For this review, take the finished solid that the model builds, in its own axes (mm). A direction names the side the tool comes from. Coordinates: 2 decimals unless noted, no trailing zeros. Write each loop counter-clockwise with the first axis right and the second up, starting at its lowest first coordinate (ties: lowest second). Pieces come first, ordered by that corner, then holes. Notation, with made-up numbers: (-34.5, 14.25) -> (19.5, 14.25) arc R17 cw to (19.5, 27.25) -> close; hole circle Ø1 at (73, 66.5). An arc over 180 degrees is marked (long way). Put each result on its own line as item: value. Start each with the question number.
Item 1: For faces 5 (the cylindrical face through (247.2, -3.47, -15.62)), 6 (the cylindrical face through (109, -6, 0)), list the 3-axis set-ups (+Z, -Z, +X, -X, +Y, -Y) from which the entire face can be reached by the end or side of a thin tool; tool diameter is ignored.
Item 2: Consider section C-C on y = -11. Give the boundary of the cut face in (x, z), and give its area (3 significant figures).
Item 3: Consider section A-A on z = 0. Give the boundary of the cut face in (x, y), and give its area (3 significant figures).
Item 4: Insertion check: P1, Ø12, axis at x = 31.5, z = 5.5, coming from the -Y side; P2, Ø8, axis at x = 91, z = 3, coming from the +Y side; P3, Ø6, axis at x = 88.5, z = 8, coming from the -Y side; P4, Ø8, axis at x = 56, y = 11.5, coming from the +Z side. Each pin has a flat end and moves straight along its axis. Give the tip position at first contact, or say it passes through.
Item 5: Consider section D-D on z = -12. Give the boundary of the cut face in (x, y).
Item 6: To check wall thickness, follow L1, parallel to X at y = 2, z = -5.5; L2, parallel to X at y = -6, z = 10.5; L3, parallel to Z at x = 84.5, y = 0. State the ranges of each line that lie inside material, in increasing order.
Item 7: Consider section B-B on x = 215. Give the boundary of the cut face in (y, z).
Item 8: The part is to be moulded in two halves that separate along X. For faces 1 (the cylindrical face through (-37.99, -1.08, -4.88)), 2 (the flat face through (-18, 3, -5)), 3 (the cylindrical face through (-27.479, -0.867, -3.905)), 4 (the flat face through (-26, 2, -4)), say which applies: +X half, -X half, draft (parallel to the pull), parting line (faces both ways), or undercut.
Autodesk Inventor part; units mm, degrees
ref_plane "accessories_l_XY" through (-38.5, 0, 0) normal (-1, 0, 0) x (0, 0, -1)
ref_plane "accessories_l_YZ" through (-38.5, 0, 0) normal (0, 0, -1) x (0, -1, 0)
ref_plane "accessories_l_ZX" through (-38.5, 0, 0) normal (0, -1, 0) x (-1, 0, 0)
sketch "Sketch_1" plane through (0, 0, 0) normal (0, 0, 1) x (1, 0, 0)
  line L0 (261, 0) -> (-48, 0)
  line L1 (-48, 0) -> (-48, 4.233)
  line L2 (-48, 4.233) -> (-47.233, 5)
  line L3 (-47.233, 5) -> (-29, 5)
  line L4 (-29, 5) -> (-29, 4)
  line L5 (-29, 4) -> (-26, 4)
  line L6 (-26, 4) -> (-26, 4.95)
  line L7 (-26, 4.95) -> (-25.45, 5.5)
  line L8 (-25.45, 5.5) -> (-18, 5.5)
  line L9 (-18, 5.5) -> (-18, 6)
  line L10 (-18, 6) -> (233, 6)
  line L11 (233, 6) -> (233, 16)
  line L12 (233, 16) -> (261, 16)
  line L13 (261, 16) -> (261, 0)
  line L14 (261, 0) -> (-48, 0)
revolve "Revolution1" add sketch "Sketch_1" angle 360 about axis through (261, 0, 0) along (1, 0, 0)
thread "Thread1"
sketch "Sketch_3" plane through (-26, 0, 0) normal (1, 0, 0) x (0, 0, -1)
  line L0 (-10, -20) -> (10, -20)
  line L1 (10, -20) -> (10, 20)
  line L2 (10, 20) -> (-10, 20)
  line L3 (-10, 20) -> (-10, -20)
  line L4 (-5, -10) -> (5, -10)
  line L5 (5, -10) -> (5, 10)
  line L6 (5, 10) -> (-5, 10)
  line L7 (-5, 10) -> (-5, -10)
extrude "Extrusion1" cut sketch "Sketch_3" along normal blind 6
ref_plane "accessories_l_XY" through (-38.5, 0, 0) normal (-1, 0, 0) x (0, 0, -1)
ref_plane "accessories_l_YZ" through (-38.5, 0, 0) normal (0, 0, -1) x (0, -1, 0)
ref_plane "accessories_l_ZX" through (-38.5, 0, 0) normal (0, -1, 0) x (-1, 0, 0)
ref_plane "rod_XY" through (0, 0, 0) normal (1, 0, 0) x (0, 0, -1)
ref_plane "rod_YZ" through (0, 0, 0) normal (0, 0, -1) x (0, 1, 0)
ref_plane "rod_ZX" through (0, 0, 0) normal (0, 1, 0) x (1, 0, 0)
properties part number "32121200-s3"
Return value:
1. face 5: +X, -X
1. face 6: -X
2. outline: (233, -11.62) -> (261, -11.62) -> (261, 11.62) -> (233, 11.62) -> close
2. area: 651 mm^2
3. outline: (-48, -4.23) -> (-47.23, -5) -> (-29, -5) -> (-29, -4) -> (-26, -4) -> (-26, -4.95) -> (-25.45, -5.5) -> (-18, -5.5) -> (-18, -6) -> (233, -6) -> (233, -16) -> (261, -16) -> (261, 16) -> (233, 16) -> (233, 6) -> (-18, 6) -> (-18, 5.5) -> (-25.45, 5.5) -> (-26, 4.95) -> (-26, 4) -> (-29, 4) -> (-29, 5) -> (-47.23, 5) -> (-48, 4.23) -> close
3. area: 4,210 mm^2
4. P1: y = -6
4. P2: y = 6
4. P3: y = -3.32
4. P4: through
5. outline: (233, -10.58) -> (261, -10.58) -> (261, 10.58) -> (233, 10.58) -> close
6. L1: -18 to 261
6. L2: 233 to 261
6. L3: -6 to 6
7. outline: circle Ø12 at (0, 0)
8. face 1: draft
8. face 2: -X half
8. face 3: undercut
8. face 4: undercut
